from build123d import *

# Parameters (mm, degrees)
SKETCH1_W           = 48
SKETCH1_H           = 52
SKETCH1_W_2         = 45
SKETCH1_H_2         = 49
BOSS_EXTRUDE1_DEPTH = 25
SKETCH2_W           = 6
SKETCH2_H           = 6
BOSS_EXTRUDE2_DEPTH = 15
SKETCH3_R           = 1
CUT_EXTRUDE1_DEPTH  = 10
SKETCH4_W           = 48
SKETCH4_H           = 52
BOSS_EXTRUDE3_DEPTH = 3
SKETCH5_W           = 25
SKETCH5_H           = 5
CUT_EXTRUDE2_DEPTH  = 3
SKETCH6_W           = 20
SKETCH6_H           = 5
CUT_EXTRUDE3_DEPTH  = 3
SKETCH7_W           = 20
SKETCH7_H           = 5
CUT_EXTRUDE4_DEPTH  = 3


with BuildPart() as part:
    # Sketch1 → Boss-Extrude1 (new body)
    with BuildSketch(Plane(origin=(0, 0, 0), x_dir=(1, 0, 0), z_dir=(0, 1, 0))):
        Rectangle(SKETCH1_W, SKETCH1_H)
        Rectangle(SKETCH1_W_2, SKETCH1_H_2, mode=Mode.SUBTRACT)
    extrude(amount=BOSS_EXTRUDE1_DEPTH)

    # Sketch2 → Boss-Extrude2 (add)
    with BuildSketch(Plane(origin=(0, 0, 0), x_dir=(1, 0, 0), z_dir=(0, 1, 0))):
        with Locations((-19.5, 21.5)):
            Rectangle(SKETCH2_W, SKETCH2_H)
        with Locations((19.5, 21.5)):
            Rectangle(SKETCH2_W, SKETCH2_H)
        with Locations((19.5, -21.5)):
            Rectangle(SKETCH2_W, SKETCH2_H)
        with Locations((-19.5, -21.5)):
            Rectangle(SKETCH2_W, SKETCH2_H)
    extrude(amount=BOSS_EXTRUDE2_DEPTH)

    # Sketch3 → Cut-Extrude1 (cut)
    with BuildSketch(Plane(origin=(0, 0, 0), x_dir=(1, 0, 0), z_dir=(0, 1, 0))):
        with Locations(Location((-18.75, 20.623770818, 0), (0, 0, 270))):
            Circle(SKETCH3_R)
        with Locations(Location((18.75, 20.623770818, 0), (0, 0, 90))):
            Circle(SKETCH3_R)
        with Locations(Location((18.75, -20.876229182, 0), (0, 0, 270))):
            Circle(SKETCH3_R)
        with Locations(Location((-18.75, -20.876229182, 0), (0, 0, 90))):
            Circle(SKETCH3_R)
    extrude(amount=CUT_EXTRUDE1_DEPTH, mode=Mode.SUBTRACT)

    # Sketch4 → Boss-Extrude3 (add)
    with BuildSketch(Plane(origin=(0, 25, 0), x_dir=(1, 0, 0), z_dir=(0, 1, 0))):
        Rectangle(SKETCH4_W, SKETCH4_H)
    extrude(amount=BOSS_EXTRUDE3_DEPTH)

    # Sketch5 → Cut-Extrude2 (cut)
    with BuildSketch(Plane.XY.offset(26)):
        with Locations((-0.148610248, 2.5)):
            Rectangle(SKETCH5_W, SKETCH5_H)
    extrude(amount=-CUT_EXTRUDE2_DEPTH, mode=Mode.SUBTRACT)

    # Sketch6 → Cut-Extrude3 (cut)
    with BuildSketch(Plane(origin=(24, 0, 0), x_dir=(0, 0, -1), z_dir=(1, 0, 0))):
        with Locations((8.266776226, 2.5)):
            Rectangle(SKETCH6_W, SKETCH6_H)
    extrude(amount=-CUT_EXTRUDE3_DEPTH, mode=Mode.SUBTRACT)

    # Sketch7 → Cut-Extrude4 (cut)
    with BuildSketch(Plane.ZY.offset(24)):
        with Locations((8.18424176, 2.5)):
            Rectangle(SKETCH7_W, SKETCH7_H)
    extrude(amount=-CUT_EXTRUDE4_DEPTH, mode=Mode.SUBTRACT)


solid = part.part
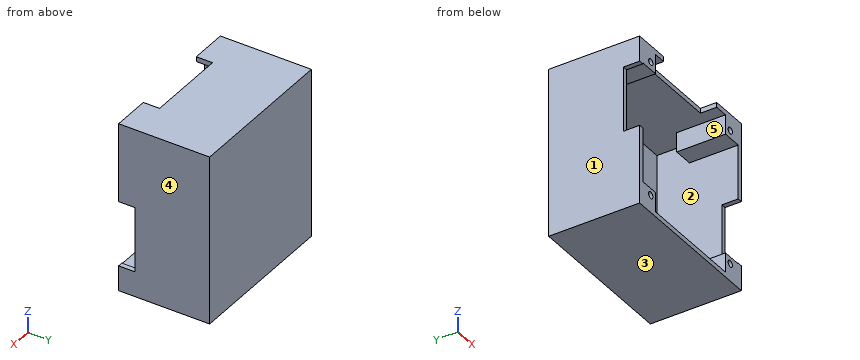
Check sheet for the modelled part. Datum: model origin and axes. Units: mm. Face numbers are marked on the shaded views. A direction names the side the tool comes from. Give positions to 0.01 mm unless a question says otherwise; leave off trailing zeros. Loops run counter-clockwise (first coordinate to the right, second up) from the corner with the lowest first, then second, coordinate; pieces in that order, holes last. Notation, with made-up numbers: M 6,10.5 L 29,10.5 A27 ccw 29,34.5 Z; hole C -36,64 d11. An arc over 180 degrees is marked long. Answer as a JSON object with one key per item and string values. Group by question number.
Q1. Material ranges on line 1 along X through (y, z) = (15.5, -0.5); line 2 along Z through (x, y) = (7, 19.5); line 3 along Z through (x, y) = (-19, 11), recorded low to high. Write a range as [from, to].
Q2. Cross-section at B-B on z = -14. Record the cut outline in (x, y).
Q3. Release check for a two-part mould opening along X. For the marked faces 3, 4 and 5 record: released by +X, released by -X, zero draft, split by the parting line, or undercut.
Q4. Go/stop test with flat-tipped pins: P1, Ø1, axis at x = 18.5, z = -20.5, coming from the -Y side; P2, Ø13.5, axis at x = 10, z = -5, coming from the -Y side. Record where each tip stops, or that it passes through.
Q5. Access from +Z, -Z, +X, -X, +Y, -Y to the whole of each face (thin tool, end or side, straight path). Record for the marked faces 1 and 2.
Q6. Cross-section at A-A on y = 9. Record the cut outline in (x, z), then the cut area to 3 significant figures.
Q7. Cross-section at C-C on x = 18.75. Record the cut outline in (y, z).
Evaluation:
{
 "1": {"line 1": "x = [-24, -22.5], [22.5, 24]", "line 2": "z = [-26, -24.5], [24.5, 26]", "line 3": "z = [-26, -18.5], [18.5, 26]"},
 "2": {"outline": "M -24,0 L -22.5,0 L -22.5,25 L 22.5,25 L 22.5,5 L 24,5 L 24,28 L -24,28 Z"},
 "3": {"face 3": "zero draft", "face 4": "released by +X", "face 5": "undercut"},
 "4": {"P1": "stops at y = 10", "P2": "stops at y = 25"},
 "5": {"face 1": "+Z, -Z, -X, +Y, -Y", "face 2": "none"},
 "6": {"outline": "M -24,-26 L 24,-26 L 24,26 L -24,26 Z; hole M -22.5,-18.5 L -16.5,-18.5 L -16.5,-24.5 L 16.5,-24.5 L 16.5,-18.5 L 22.5,-18.5 L 22.5,18.5 L 16.5,18.5 L 16.5,24.5 L -16.5,24.5 L -16.5,18.5 L -22.5,18.5 Z; hole C -18.75,-20.62 d2; hole C -18.75,20.88 d2; hole C 18.75,-20.62 d2; hole C 18.75,20.88 d2", "area": "422 mm2"},
 "7": {"outline": "M 0,-26 L 28,-26 L 28,26 L 0,26 L 0,21.88 L 10,21.88 L 10,19.88 L 0,19.88 L 0,18.5 L 15,18.5 L 15,24.5 L 25,24.5 L 25,-24.5 L 15,-24.5 L 15,-18.5 L 0,-18.5 L 0,-19.62 L 10,-19.62 L 10,-21.62 L 0,-21.62 Z"}
}
